Geometry check sheet. Reference: the model listing, model coordinates, mm. Face numbers are marked on the shaded views. A direction names the side the tool comes from. Coordinates: 2 decimals unless noted, no trailing zeros. Loops run counter-clockwise (first coordinate to the right, second up) from the corner with the lowest first, then second, coordinate; pieces in that order, holes last. Notation, with made-up numbers: (79.5, 75) -> (117.5, 75) arc R20 cw to (117.5, 102) -> close; hole circle Ø1 at (-21.75, 86.5). An arc over 180 degrees is marked (long way). Answer as a JSON object with one key per item and string values.
from build123d import *

# Parameters (mm, degrees)
EXTRUDE_388_DEPTH      = 20
FILLET_1_R             = 2
SKETCH_6_R             = 1
CUT_EXTRUDE_1034_DEPTH = 7
CUT_EXTRUDE_1428_REACH = 45.313
SKETCH_3_W             = 16.6
SKETCH_3_H             = 3
SKETCH_2_W             = 21
SKETCH_2_H             = 1.8
CUT_EXTRUDE_1921_DEPTH = 12
SKETCH_7_W             = 16.6
SKETCH_7_H             = 2.2
CUT_EXTRUDE_1_DEPTH    = 12


with BuildPart() as part:
    # Эскиз1 → Extrude 388 (new body)
    with BuildSketch(Plane(origin=(0, 0, 0), x_dir=(1, 0, 0), z_dir=(0, 1, 0))):
        with BuildLine():
            Line((4, 0), (26, 0))
            ThreePointArc((26, 0), (28.828427125, 1.171572875), (30, 4))
            Line((30, 4), (30, 20))
            ThreePointArc((30, 20), (28.828427125, 22.828427125), (26, 24))
            Line((26, 24), (4, 24))
            ThreePointArc((4, 24), (1.171572875, 22.828427125), (0, 20))
            Line((0, 20), (0, 4))
            ThreePointArc((0, 4), (1.171572875, 1.171572875), (4, 0))
        make_face()
    extrude(amount=EXTRUDE_388_DEPTH)

    # Скругление1
    fillet_1_edges = [part.edges().sort_by_distance(p)[0] for p in [
        (1.171572875, 20, -22.828427125),
        (0, 20, -12),
        (1.171572875, 20, -1.171572875),
        (15, 20, 0),
        (28.828427125, 20, -1.171572875),
        (30, 20, -12),
        (28.828427125, 20, -22.828427125),
        (15, 20, -24),
    ]]
    fillet(fillet_1_edges, radius=FILLET_1_R)

    # Эскиз6 → Cut-Extrude 1034 (cut)
    with BuildSketch(Plane.XZ):
        with Locations(Location((4, -4, 0), (0, 0, 270))):
            Circle(SKETCH_6_R)
        with Locations(Location((26, -4, 0), (0, 0, 270))):
            Circle(SKETCH_6_R)
        with Locations(Location((26, -20, 0), (0, 0, 270))):
            Circle(SKETCH_6_R)
        with Locations(Location((4, -20, 0), (0, 0, 270))):
            Circle(SKETCH_6_R)
    extrude(amount=-CUT_EXTRUDE_1034_DEPTH, mode=Mode.SUBTRACT)

    # Эскиз3 → Cut-Extrude 1428 (cut, up to next)
    with BuildSketch(Plane(origin=(0, 20, 0), x_dir=(1, 0, 0), z_dir=(0, 1, 0)), mode=Mode.PRIVATE) as cut_extrude_1428_sk1:
        with Locations((15, 9.9)):
            Rectangle(SKETCH_3_W, SKETCH_3_H)
    cut_extrude_1428_tool1 = extrude(cut_extrude_1428_sk1.sketch, amount=-CUT_EXTRUDE_1428_REACH, mode=Mode.PRIVATE) & part.part
    add(cut_extrude_1428_tool1.solids().sort_by_distance((15, 20, -9.9))[0], mode=Mode.SUBTRACT)

    # Эскиз2 → Cut-Extrude 1921 (cut)
    with BuildSketch(Plane(origin=(0, 20, 0), x_dir=(1, 0, 0), z_dir=(0, 1, 0))):
        with Locations((15, 11.9)):
            Rectangle(SKETCH_2_W, SKETCH_2_H)
    extrude(amount=-CUT_EXTRUDE_1921_DEPTH, mode=Mode.SUBTRACT)

    # Эскиз7 → Вырез-Вытянуть1 (cut)
    with BuildSketch(Plane(origin=(0, 20, 0), x_dir=(1, 0, 0), z_dir=(0, 1, 0))):
        with Locations((15, 13.9)):
            Rectangle(SKETCH_7_W, SKETCH_7_H)
    extrude(amount=-CUT_EXTRUDE_1_DEPTH, mode=Mode.SUBTRACT)


solid = part.part
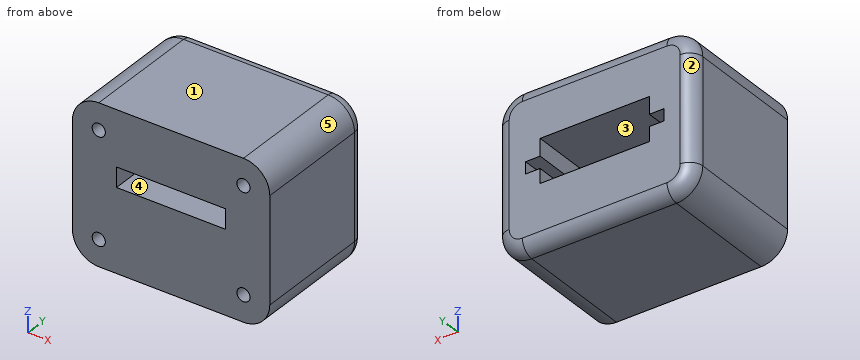
1. Mould release check, pull along X, two halves, no side actions. Record for the marked faces 1, 2 and 3: released by +X, released by -X, zero draft, split by the parting line, or undercut.
Evaluation:
{"face 1": "zero draft", "face 2": "released by -X", "face 3": "undercut"}
2. Section check B-B, the plane z = -10. Record the boundary of the cut face in (x, y), then the cut area to 3 significant figures.
Evaluation:
{"outline": "(0, 0) -> (6.7, 0) -> (6.7, 20) -> (2, 20) arc R2 ccw to (0, 18) -> close; (23.3, 0) -> (30, 0) -> (30, 18) arc R2 ccw to (28, 20) -> (23.3, 20) -> close", "area": "266 mm^2"}
3. Tool access check on the marked faces 4 and 5. Record the directions out of +Z, -Z, +X, -X, +Y, -Y that give a thin tool (end or side, any length) a straight path to the whole face; none if there is none.
Evaluation:
{"face 4": "+Y, -Y", "face 5": "+Z, +X, +Y, -Y"}
4. Section check A-A, the plane x = 18.5. Record the boundary of the cut face in (y, z), then the cut area to 3 significant figures.
Evaluation:
{"outline": "(0, -24) -> (18, -24) arc R2 ccw to (20, -22) -> (20, -15) -> (8, -15) -> (8, -11.4) -> (0, -11.4) -> close; (0, -8.4) -> (20, -8.4) -> (20, -2) arc R2 ccw to (18, 0) -> (0, 0) -> close", "area": "375 mm^2"}
5. Thickness scan on probe 1 along X at (y, z) = (4.25, -20); probe 2 along Z at (x, y) = (7.25, 17.25); probe 3 along Z at (x, y) = (13.25, 18.75). Record the ranges inside material, lowest first. Write a range as from..to.
Evaluation:
{"probe 1": "x = 0..3, 5..25, 27..30", "probe 2": "z = -24..-15, -8.4..0", "probe 3": "z = -23.85..-15, -8.4..-0.15"}
6. Section check D-D, the plane y = 2.25. Record the boundary of the cut face in (x, z), then the cut area to 3 significant figures.
Evaluation:
{"outline": "(0, -20) arc R4 ccw to (4, -24) -> (26, -24) arc R4 ccw to (30, -20) -> (30, -4) arc R4 ccw to (26, 0) -> (4, 0) arc R4 ccw to (0, -4) -> close; hole circle Ø2 at (4, -20); hole circle Ø2 at (4, -4); hole (6.7, -11.4) -> (23.3, -11.4) -> (23.3, -8.4) -> (6.7, -8.4) -> close; hole circle Ø2 at (26, -20); hole circle Ø2 at (26, -4)", "area": "644 mm^2"}
7. Section check C-C, the plane y = 11.5. Record the boundary of the cut face in (x, z), then the cut area to 3 significant figures.
Evaluation:
{"outline": "(0, -20) arc R4 ccw to (4, -24) -> (26, -24) arc R4 ccw to (30, -20) -> (30, -4) arc R4 ccw to (26, 0) -> (4, 0) arc R4 ccw to (0, -4) -> close; hole (4.5, -12.8) -> (6.7, -12.8) -> (6.7, -15) -> (23.3, -15) -> (23.3, -12.8) -> (25.5, -12.8) -> (25.5, -11) -> (23.3, -11) -> (23.3, -8.4) -> (6.7, -8.4) -> (6.7, -11) -> (4.5, -11) -> close", "area": "589 mm^2"}
8. Depth check by flat-ended pin: P1, Ø1.2, axis at x = 18, z = -13.5, coming from the +Y side; P2, Ø1.2, axis at x = 4, z = -4, coming from the -Y side. Enter the tip coordinate at first touch or a pass-through.
Evaluation:
{"P1": "stops at y = 8", "P2": "stops at y = 7"}
